```python
from build123d import *


with BuildPart() as f1:
    # F0 (on Front) → F1 (revolve)
    with BuildSketch(Plane.XZ):
        with BuildLine():
            Line((-16.637, 41.275), (-19.812, 41.275))
            Line((-19.812, 41.275), (-19.812, -34.925))
            Line((-19.812, -34.925), (-16.637, -34.925))
            Line((-16.637, -34.925), (-16.637, -1.5875))
            ThreePointArc((-16.637, -1.5875), (-16.172032, -0.464968), (-15.0495, 0))
            Line((-15.0495, 0), (-12, 0))
            Line((-12, 0), (-12, 3.175))
            Line((-12, 3.175), (-7, 3.175))
            Line((-7, 3.175), (-7, 6.35))
            Line((-7, 6.35), (-15.0495, 6.35))
            ThreePointArc((-15.0495, 6.35), (-16.172032, 6.814968), (-16.637, 7.9375))
            Line((-16.637, 7.9375), (-16.637, 41.275))
        make_face()
    revolve(axis=Axis((0, 0, -3.752202), (0, 0, -1)))


solid = f1.part
```
Check sheet for the modelled part. Datum: model origin and axes. Units: mm. A direction names the side the tool comes from. Coordinates: 2 decimals unless noted, no trailing zeros. Order: outer loops, then holes, each group sorted by start corner. A loop starts at its lowest first (then second) coordinate and runs counter-clockwise, first axis right, second up. Notation, with made-up numbers: M 59.25,89 L 91.25,89 A13 ccw 91.25,108 Z; hole C 88,-19.5 d9. An arc over 180 degrees is marked long. Write each question's results on one line, items separated by ' | '. Start each with the question number.
1. Go/stop test with flat-tipped pins: P1, Ø7, axis at x = -1, y = -5.5, coming from the -Z side (3 decimals); P2, Ø4, axis at x = 13, z = -6.5, coming from the -Y side; P3, Ø22.5, axis at x = 0, y = 0, coming from the +Z side. Record where each tip stops, or that it passes through.
2. Mould release check, pull along Y, two halves, no side actions. Record for faces 1 (the face through (6.5, -3.1, 6.35)), 2 (the face through (-4.5, 16.2, 41.275)), 3 (the face through (2.579, 19.643, 2.642)): +Y half, -Y half, draft (parallel to the pull), parting line (faces both ways), or undercut.
3. Cross-section at C-C on z = -20.5. Record the cut outline in (x, y).
4. Material ranges on probe 1 along Y at (x, z) = (0, 4.1); probe 2 along Y at (x, z) = (0, 19.5); probe 3 along X at (y, z) = (-3, -11.5), recorded low to high.
5. Access from +Z, -Z, +X, -X, +Y, -Y to the whole of each face (thin tool, end or side, straight path). Record for faces 4 (the face through (2.166, 16.495, 24.84)), 5 (the face through (-6.466, -2.681, 4.785)), 6 (the face through (-5.2, -5.2, 3.175)).
Checks:
1) P1: stops at z = 3.175 | P2: stops at y = -16.48 | P3: stops at z = 6.35
2) face 1: undercut | face 2: draft | face 3: parting line
3) outline: C 0,0 d39.62; hole C 0,0 d33.27
4) probe 1: y = -19.81 to -7, 7 to 19.81 | probe 2: y = -19.81 to -16.64, 16.64 to 19.81 | probe 3: x = -19.58 to -16.36, 16.36 to 19.58
5) face 4: +Z | face 5: +Z, -Z | face 6: -Z
